```python
from build123d import *

# Parameters (mm, degrees)
CROQUIS1_R              = 1.6
SALIENTE_EXTRUIR1_DEPTH = 6
CROQUIS1_3_R            = 4
CROQUIS1_3_R_2          = 1.6
CORTAR_EXTRUIR1_DEPTH   = 4
REDONDEO1_R             = 4


with BuildPart() as part:
    # Croquis1 → Saliente-Extruir1 (new body)
    with BuildSketch(Plane(origin=(0, 0, 0), x_dir=(1, 0, 0), z_dir=(0, 1, 0))):
        with BuildLine():
            Line((57, 37.7), (-57, 37.7))
            ThreePointArc((-57, 37.7), (-59.828427125, 36.528427125), (-61, 33.7))
            Line((-61, 33.7), (-61, -33.7))
            ThreePointArc((-61, -33.7), (-59.828427125, -36.528427125), (-57, -37.7))
            Line((-57, -37.7), (57, -37.7))
            ThreePointArc((57, -37.7), (59.828427125, -36.528427125), (61, -33.7))
            Line((61, -33.7), (61, 33.7))
            ThreePointArc((61, 33.7), (59.828427125, 36.528427125), (57, 37.7))
        make_face()
        with BuildLine():
            Line((-57, 30.871572875), (-37, 10.871572875))
            Line((-37, 10.871572875), (-37, 8.7))
            ThreePointArc((-37, 8.7), (-36.327649298, 6.195713365), (-34.491419379, 4.36493028))
            ThreePointArc((-34.491419379, 4.36493028), (-31.965559308, 0), (-34.491419379, -4.36493028))
            ThreePointArc((-34.491419379, -4.36493028), (-36.327649298, -6.195713365), (-37, -8.7))
            Line((-37, -8.7), (-37, -10.871572875))
            Line((-37, -10.871572875), (-57, -30.871572875))
            Line((-57, -30.871572875), (-57, 30.871572875))
        make_face(mode=Mode.SUBTRACT)
        with BuildLine():
            Line((-54.171572875, -33.7), (-34.171572875, -13.7))
            Line((-34.171572875, -13.7), (-32, -13.7))
            ThreePointArc((-32, -13.7), (-28.464466094, -12.235533906), (-27, -8.7))
            Line((-27, -8.7), (-27, -5.7))
            Line((-27, -5.7), (27, -5.7))
            Line((27, -5.7), (27, -8.7))
            ThreePointArc((27, -8.7), (28.464466094, -12.235533906), (32, -13.7))
            Line((32, -13.7), (34.171572875, -13.7))
            Line((34.171572875, -13.7), (54.171572875, -33.7))
            Line((54.171572875, -33.7), (-54.171572875, -33.7))
        make_face(mode=Mode.SUBTRACT)
        with BuildLine():
            Line((57, -30.871572875), (37, -10.871572875))
            Line((37, -10.871572875), (37, -8.7))
            ThreePointArc((37, -8.7), (36.327649298, -6.195713365), (34.491419379, -4.36493028))
            ThreePointArc((34.491419379, -4.36493028), (31.965559308, 0), (34.491419379, 4.36493028))
            ThreePointArc((34.491419379, 4.36493028), (36.327649298, 6.195713365), (37, 8.7))
            Line((37, 8.7), (37, 10.871572875))
            Line((37, 10.871572875), (57, 30.871572875))
            Line((57, 30.871572875), (57, -30.871572875))
        make_face(mode=Mode.SUBTRACT)
        with BuildLine():
            Line((54.171572875, 33.7), (34.171572875, 13.7))
            Line((34.171572875, 13.7), (32, 13.7))
            ThreePointArc((32, 13.7), (28.464466094, 12.235533906), (27, 8.7))
            Line((27, 8.7), (27, 5.7))
            Line((27, 5.7), (-27, 5.7))
            Line((-27, 5.7), (-27, 8.7))
            ThreePointArc((-27, 8.7), (-28.464466094, 12.235533906), (-32, 13.7))
            Line((-32, 13.7), (-34.171572875, 13.7))
            Line((-34.171572875, 13.7), (-54.171572875, 33.7))
            Line((-54.171572875, 33.7), (54.171572875, 33.7))
        make_face(mode=Mode.SUBTRACT)
        with BuildLine():
            Line((-27, 3.7), (27, 3.7))
            ThreePointArc((27, 3.7), (28.961617728, 0), (27, -3.7))
            Line((27, -3.7), (-27, -3.7))
            ThreePointArc((-27, -3.7), (-28.961617728, 0), (-27, 3.7))
        make_face(mode=Mode.SUBTRACT)
        with Locations((-32, 8.7)):
            Circle(CROQUIS1_R, mode=Mode.SUBTRACT)
        with Locations((32, 8.7)):
            Circle(CROQUIS1_R, mode=Mode.SUBTRACT)
        with Locations((32, -8.7)):
            Circle(CROQUIS1_R, mode=Mode.SUBTRACT)
        with Locations((-32, -8.7)):
            Circle(CROQUIS1_R, mode=Mode.SUBTRACT)
    extrude(amount=SALIENTE_EXTRUIR1_DEPTH)

    # Croquis1_3 → Cortar-Extruir1 (cut)
    with BuildSketch(Plane(origin=(0, 0, 0), x_dir=(1, 0, 0), z_dir=(0, 1, 0))):
        with Locations((-32, -8.7)):
            Circle(CROQUIS1_3_R)
        with Locations((-32, -8.7)):
            Circle(CROQUIS1_3_R_2, mode=Mode.SUBTRACT)
        with Locations((-32, 8.7)):
            Circle(CROQUIS1_3_R)
        with Locations((-32, 8.7)):
            Circle(CROQUIS1_3_R_2, mode=Mode.SUBTRACT)
        with Locations((32, 8.7)):
            Circle(CROQUIS1_3_R)
        with Locations((32, 8.7)):
            Circle(CROQUIS1_3_R_2, mode=Mode.SUBTRACT)
        with Locations((32, -8.7)):
            Circle(CROQUIS1_3_R)
        with Locations((32, -8.7)):
            Circle(CROQUIS1_3_R_2, mode=Mode.SUBTRACT)
    extrude(amount=CORTAR_EXTRUIR1_DEPTH, mode=Mode.SUBTRACT)

    # Redondeo1
    redondeo1_edges = [part.edges().sort_by_distance(p)[0] for p in [
        (27, 3, -5.7),
        (27, 3, 5.7),
        (-27, 3, -5.7),
        (-27, 3, 5.7),
    ]]
    fillet(redondeo1_edges, radius=REDONDEO1_R)


solid = part.part
```
Verification items for the finished model (mm, model axes). A direction names the side the tool comes from. Coordinates: 2 decimals unless noted, no trailing zeros. Write each loop counter-clockwise with the first axis right and the second up, starting at its lowest first coordinate (ties: lowest second). Pieces come first, ordered by that corner, then holes. Notation, with made-up numbers: M 50.25,3 L 103.25,3 A23 ccw 103.25,41 Z; hole C 49,45 d5. An arc over 180 degrees is marked long. One line per item, written item: value.
Item 1: Section check C-C, the plane y = 1.75. State how many separate pieces and enclosed holes the cut face has, plus the area to 3 significant figures.
Check sheet entries:
separate pieces: 1
enclosed holes: 9
area: 2,400 mm^2
Item 2: Mould release check, pull along X, two halves, no side actions. Record for faces 1 (the cylindrical face through (-59.797, 2.958, -36.559)), 2 (the cylindrical face through (31.966, 2.958, 0.074)), 3 (the flat face through (-30, 4, -9)): pulls with the +X half, pulls with the -X half, needs draft (parallel to the pull), parting line crosses it, or undercut.
Check sheet entries:
face 1: pulls with the -X half
face 2: undercut
face 3: undercut
Item 3: Access from +Z, -Z, +X, -X, +Y, -Y to the whole of each face (thin tool, end or side, straight path). Record for faces 4 (the cylindrical face through (-59.859, 2.958, 36.497)), 5 (the flat face through (34, 4, -9)), 6 (the flat face through (47.14, 2.96, 21.01)).
Check sheet entries:
face 4: +Z, -X, +Y, -Y
face 5: -Y
face 6: +Y, -Y
Item 4: Scan lines: line 1 along Z through (x, y) = (14.5, 0.75); line 2 along X through (y, z) = (2, 0.5); line 3 along Z through (x, y) = (54, 3). Record each from-to range of solid material in increasing order.
Check sheet entries:
line 1: z = -37.7 to -33.7, -5.7 to -3.7, 3.7 to 5.7, 33.7 to 37.7
line 2: x = -61 to -57, -31.99 to -28.93, 28.93 to 31.99, 57 to 61
line 3: z = -37.7 to -33.7, -33.53 to -27.87, 27.87 to 33.53, 33.7 to 37.7
Item 5: Gauge pin test, flat ends, axial feed: pin 1 Ø1.9 at (x, z) = (32, -8.7) entering from +Y (3 decimals); pin 2 Ø4 at (x, z) = (-32, -8.7) entering from -Y. Record the tip position at first contact, or that the pin passes through.
Check sheet entries:
pin 1: passes through
pin 2: stops at y = 4
Item 6: Section check B-B, the plane z = 1.5. Record the boundary of the cut face in (x, y), plus the area to 3 significant figures.
Check sheet entries:
outline: M -61,0 L -57,0 L -57,6 L -61,6 Z; M -32.19,0 L -28.7,0 L -28.7,6 L -32.19,6 Z; M 28.7,0 L 32.19,0 L 32.19,6 L 28.7,6 Z; M 57,0 L 61,0 L 61,6 L 57,6 Z
area: 89.9 mm^2
Item 7: Section check A-A, the plane x = -1. Record the boundary of the cut face in (y, z).
Check sheet entries:
outline: M 0,-37.7 L 6,-37.7 L 6,-33.7 L 0,-33.7 Z; M 0,-5.7 L 6,-5.7 L 6,-3.7 L 0,-3.7 Z; M 0,3.7 L 6,3.7 L 6,5.7 L 0,5.7 Z; M 0,33.7 L 6,33.7 L 6,37.7 L 0,37.7 Z
